The model under review builds one solid part; all positions refer to its coordinate system, in mm. Give positions to 0.01 mm unless a question says otherwise; leave off trailing zeros. Loops run counter-clockwise (first coordinate to the right, second up) from the corner with the lowest first, then second, coordinate; pieces in that order, holes last. Notation, with made-up numbers: M 40,-39 L 86,-39 A16 ccw 86,-27 Z; hole C 67.5,38.5 d3. An arc over 180 degrees is marked long. Put each result on its own line as item: value. Start each with the question number.
from build123d import *

# Parameters (mm, degrees)
SKETCH1_R           = 88.9
SKETCH1_R_2         = 63.5
BOSS_EXTRUDE1_DEPTH = 25.4
FILLET1_R           = 1.27


with BuildPart() as part:
    # Sketch1 → Boss-Extrude1 (new, symmetric)
    with BuildSketch(Plane(origin=(0, 0, 0), x_dir=(0, 0, -1), z_dir=(1, 0, 0))):
        Circle(SKETCH1_R)
        Circle(SKETCH1_R_2, mode=Mode.SUBTRACT)
    extrude(amount=BOSS_EXTRUDE1_DEPTH, both=True)

    # Fillet1
    fillet1_edges = [part.edges().sort_by_distance(p)[0] for p in [
        (-25.4, 0, 88.9),
        (25.4, 0, 88.9),
        (25.4, 0, 63.5),
    ]]
    fillet(fillet1_edges, radius=FILLET1_R)


solid = part.part
(1) Draft analysis for pull direction Y (two halves, no side actions). For faces 1 (the cylindrical face through (-0.98, -61.99, 13.77)), 2 (the cylindrical face through (0.338, 26.703, -84.795)), 3 (the flat face through (-25.4, 26.4, -58)), state which applies: +Y half, -Y half, draft (parallel to the pull), parting line (faces both ways), or undercut.
(2) We need section A-A, the plane z = 0. Write out the cut boundary in (x, y), plus the area to 3 significant figures.
(3) To check wall thickness, follow L1, parallel to Y at x = 12, z = 0; L2, parallel to Z at x = -12.5, y = 16; L3, parallel to Z at x = 7, y = 30.5. State the ranges of each line that lie inside material, in increasing order. Write a range as [from, to].
(4) We need section C-C, the plane x = -2.5. Write out the cut boundary in (y, z).
(5) Insertion check: pin 1 (2 mm diameter, centred on x = 10.5, z = -4.5, fed in from -Y); pin 2 (8 mm diameter, centred on x = 14, y = 16.5, fed in from +Z); pin 3 (2 mm diameter, centred on x = -12, z = 25.5, fed in from -Y). Each pin has a flat end and moves straight along its axis. Give the tip position at first contact, or say it passes through.
Check sheet entries:
1. face 1: undercut
1. face 2: parting line
1. face 3: draft
2. outline: M -25.4,-87.63 A1.27 ccw -24.13,-88.9 L 24.13,-88.9 A1.27 ccw 25.4,-87.63 L 25.4,-64.77 A1.27 ccw 24.13,-63.5 L -25.4,-63.5 Z; M -25.4,63.5 L 24.13,63.5 A1.27 ccw 25.4,64.77 L 25.4,87.63 A1.27 ccw 24.13,88.9 L -24.13,88.9 A1.27 ccw -25.4,87.63 Z
2. area: 2,580 mm²
3. L1: y = [-88.9, -63.5], [63.5, 88.9]
3. L2: z = [-87.45, -61.45], [61.45, 87.45]
3. L3: z = [-83.5, -55.7], [55.7, 83.5]
4. outline: C 0,0 d177.8; hole C 0,0 d127
5. pin 1: stops at y = -88.83
5. pin 2: stops at z = 88.02
5. pin 3: stops at y = -85.46
